from build123d import *

# Parameters (mm, degrees)
F1_DEPTH = 25
F2_R     = 6.331158
F3_DEPTH = 55
F4_R     = 4.545947
F5_DEPTH = 51.663236
F6_R     = 3.2686
F7_DEPTH = 55.001


with BuildPart() as f1:
    # F0 (on Top) → F1 (new body)
    with BuildSketch(Plane.XY):
        Polygon((23.736702, 9.494681), (0, 0), (-11.170213, -3.071809), (-27.646277, -3.071809), (-51.662236, 0), (-51.662236, -6.143617), (-40.212769, -30.438831), (-29.461436, -31.695481), (-18.710107, -32.95213), (6.143617, -32.95213), (27.872912, -14.656438), (32.393619, 20.94415), (14.800533, 23.178192), align=None)
    extrude(amount=F1_DEPTH)

    # F2 (on Right) → F3 (join)
    with BuildSketch(Plane.YZ):
        with Locations((10.890958, 16.476065)):
            Circle(F2_R)
    extrude(amount=F3_DEPTH)

    # F4 (on Right) → F5 (cut, through all)
    with BuildSketch(Plane.YZ):
        with Locations((10.890957, 16.75532)):
            Circle(F4_R)
    extrude(amount=-F5_DEPTH, mode=Mode.SUBTRACT)

    # F6 (on Right) → F7 (cut, through all)
    with BuildSketch(Plane.YZ):
        with Locations((11.170213, 16.75532)):
            Circle(F6_R)
    extrude(amount=F7_DEPTH, mode=Mode.SUBTRACT)


solid = f1.part
Geometry: final body of the model. Coordinates: model frame, mm. A direction names the side the tool comes from. Give positions to 0.01 mm unless a question says otherwise; leave off trailing zeros. Loops run counter-clockwise (first coordinate to the right, second up) from the corner with the lowest first, then second, coordinate; pieces in that order, holes last. Notation, with made-up numbers: (42.5, 80) - (50.5, 80) arc R23 cw to (50.5, 119) - close; hole circle Ø8 at (-14, 32.25). An arc over 180 degrees is marked (long way). Answer as CSV lines item,"result". Start each with the question number.
1. Section D-D, the plane z = 7.5. Return loops of the section in (x, y).
2. Section B-B, the plane x = 1.5. Return loops of the section in (y, z), plus the area to 3 significant figures.
3. Reachability of faces 1 (the face through (-19, -3.072, 12)), 2 (the face through (23.72, 22.046, 12.325)), 3 (the face through (42.445, 4.566, 16.754)) from +Z, -Z, +X, -X, +Y, -Y: full face, straight path, thin tool, end or side. Return the list, or none.
4. Section A-A, the plane z = 14.75. Return loops of the section in (x, y).
5. Ray query, L1, parallel to Y at x = -14.5, z = 18.75; L2, parallel to Z at x = 13, y = 12.5; L3, parallel to X at y = 5, z = 21.75. Return the intervals inside material, ascending.
6. Section C-C, the plane y = -1. Return loops of the section in (x, z), plus the area to 3 significant figures.
7. Pin query (flat end, axial travel): P1, Ø1.5, axis at x = 40.5, z = 21, coming from the -Y side; P2, Ø6, axis at y = 11.17, z = 16.76, coming from the +X side; P3, Ø13, axis at x = -18.5, z = 12.5, coming from the +Y side; P4, Ø2, axis at x = 9, z = 10.5, coming from the +Y side. Return the tip coordinate at first contact, or that it passes through.
8. Draft query along Z for faces 4 (the face through (27.12, 12.93, 19.51)), 5 (the face through (0, 9, 14)), 6 (the face through (-10, -11, 25)). Return one class per face: released by +Z, released by -Z, zero draft, split by the parting line, or undercut.
Answers:
1,outline,"(-51.66, -6.14) - (-40.21, -30.44) - (-18.71, -32.95) - (6.14, -32.95) - (27.87, -14.66) - (32.39, 20.94) - (14.8, 23.18) - (23.74, 9.49) - (0, 0) - (-11.17, -3.07) - (-27.65, -3.07) - (-51.66, 0) - close"
2,outline,"(-32.95, 0) - (0.6, 0) - (0.6, 25) - (-32.95, 25) - close; circle Ø12.66 at (10.89, 16.48); hole circle Ø6.54 at (11.17, 16.76)"
2,area,"931 mm2"
3,face 1,"+Z, -Z, +Y"
3,face 2,"+Z, -Z, +X, +Y"
3,face 3,"+X"
4,outline,"(-51.66, -6.14) - (-40.21, -30.44) - (-18.71, -32.95) - (6.14, -32.95) - (27.87, -14.66) - (30.34, 4.8) - (55, 4.8) - (55, 8.59) - (0, 8.59) - (0, 4.8) - (12, 4.8) - (0, 0) - (-11.17, -3.07) - (-27.65, -3.07) - (-51.66, 0) - close; (0, 13.75) - (55, 13.75) - (55, 16.98) - (31.89, 16.98) - (32.39, 20.94) - (14.8, 23.18) - (18.85, 16.98) - (0, 16.98) - close"
5,L1,"y = -32.95 to -3.07"
5,L2,"z = 10.35 to 13.77, 19.74 to 22.6"
5,L3,"x = 12.5 to 30.37"
6,outline,"(-51.66, 0) - (-43.84, 0) - (-43.84, 25) - (-51.66, 25) - close; (-3.64, 0) - (29.61, 0) - (29.61, 25) - (-3.64, 25) - close"
6,area,"1,030 mm2"
7,P1,"stops at y = 5.81"
7,P2,"passes through"
7,P3,"stops at y = -3.07"
7,P4,"stops at y = 14.81"
8,face 4,"undercut"
8,face 5,"zero draft"
8,face 6,"released by +Z"
